Autodesk Inventor part; units mm, degrees
ref_plane "YZ Plane" through (0, 0, 0) normal (1, 0, 0) x (0, 1, 0)
ref_plane "XZ Plane" through (0, 0, 0) normal (0, 1, 0) x (-1, 0, 0)
ref_plane "XY Plane" through (0, 0, 0) normal (0, 0, 1) x (1, 0, 0)
sketch "Sketch1" plane through (0, 0, 0) normal (0, 0, 1) x (1, 0, 0)
  line L0 (0, 0) -> (34.66, 0)
  line L1 (34.66, 0) -> (34.66, -34.66)
  line L2 (34.66, -34.66) -> (0, -34.66)
  line L3 (0, -34.66) -> (0, 0)
  dimension "d0" = 34.66
  dimension "d1" = 34.66
extrude "Extrusion1" add sketch "Sketch1" along normal blind 21.5
sketch "Sketch2" plane through (0, 0, 21.5) normal (0, 0, 1) x (1, 0, 0)
  line L0 (0, 0) -> (0, -34.66)
  line L1 (3, -3) -> (31.66, -3)
  line L2 (31.66, -3) -> (31.66, -31.66)
  line L3 (31.66, -31.66) -> (3, -31.66)
  line L4 (3, -31.66) -> (3, -3)
  line L5 (34.66, 0) -> (0, 0)
  line L6 (0, -34.66) -> (34.66, -34.66)
  line L7 (34.66, 0) -> (34.66, -34.66)
  dimension "d8" = 3
  dimension "d9" = 3
  dimension "d10" = 3
  dimension "d11" = 3
extrude "Extrusion2" cut sketch "Sketch2" against normal blind 3.5 contours L1 L2 L3 L4
sketch "Sketch3" plane through (0, 0, 18) normal (0, 0, 1) x (1, 0, 0)
  line L0 (12.08, -3) -> (12.08, -6)
  line L1 (12.08, -6) -> (22.58, -6)
  line L2 (22.58, -6) -> (22.58, -3)
  line L3 (12.08, -3) -> (22.58, -3)
  line L4 (3, -3) -> (31.66, -3)
  line L5 (3, -31.66) -> (3, -3)
  line L6 (31.66, -3) -> (31.66, -31.66)
  line L7 (31.66, -31.66) -> (3, -31.66)
  point P0 (0, 0)
  dimension "d18" = 9.08
  dimension "d19" = 9.08
  dimension "d20" = 3
  dimension "d21" = 28.66
extrude "Extrusion3" cut sketch "Sketch3" against normal blind 19 contours L3 L2 L1 L0
properties part number "Pantalla"
Here's how the part is built. I have some questions about the finished solid (model axes, mm). A direction names the side the tool comes from. Round coordinates to 2 decimals unless told otherwise and drop trailing zeros. Order: outer loops, then holes, each group sorted by start corner. A loop starts at its lowest first (then second) coordinate and runs counter-clockwise, first axis right, second up. Notation, with made-up numbers: (-2.5, 50) -> (23.5, 50) arc R11 cw to (23.5, 66) -> close; hole circle Ø2 at (-1.5, -29.75). An arc over 180 degrees is marked (long way). Use a Markdown table: item, result. Add a question column.
(1) Suppose I cut it at B-B, the plane x = 13. Please give me the cut outline in (y, z).
(2) Suppose I cut it at D-D, the plane y = -26. Please give me the cut outline in (x, z).
(3) If we mould it in two halves opening along Y, with no side actions, what happens to faces 1 (the face through (22.58, -5, 9)), 2 (the face through (17, 0, 11)), 3 (the face through (34.66, -17, 11))? For each: released by +Y, released by -Y, zero draft, split by the parting line, or undercut.
(4) I need wall thicknesses on line 1 along X through (y, z) = (-5, 3); line 2 along Y through (x, z) = (20, 8.25); line 3 along Z through (x, y) = (11, -4). Which ranges of each line are inside material? Lowest first, please.
(5) For faces 4 (the face through (0, -18, 11)), 5 (the face through (17, -6, 9)), 6 (the face through (31.66, -17, 20)), which set-ups out of +Z, -Z, +X, -X, +Y, -Y let a thin tool reach every point of the face, with its end or its side?
(6) Suppose I cut it at C-C, the plane z = 9.75. Please give me the cut outline in (x, y).
(7) Suppose I cut it at A-A, the plane y = -5. Please give me the cut outline in (x, z).
(8) For pin 1 Ø1 at (x, y) = (12.5, -8.5) entering from +Z, with a flat end and sliding along its axis, tell me the tip position at first contact or that it passes through.
Verdict:
| question | item | result |
|---|---|---|
| 1 | outline | (-34.66, 0) -> (-6, 0) -> (-6, 18) -> (-31.66, 18) -> (-31.66, 21.5) -> (-34.66, 21.5) -> close; (-3, 0) -> (0, 0) -> (0, 21.5) -> (-3, 21.5) -> close |
| 2 | outline | (0, 0) -> (34.66, 0) -> (34.66, 21.5) -> (31.66, 21.5) -> (31.66, 18) -> (3, 18) -> (3, 21.5) -> (0, 21.5) -> close |
| 3 | face 1 | undercut |
| 3 | face 2 | released by +Y |
| 3 | face 3 | zero draft |
| 4 | line 1 | 0 to 12.08, 22.58 to 34.66 |
| 4 | line 2 | -34.66 to -6, -3 to 0 |
| 4 | line 3 | 0 to 18 |
| 5 | face 4 | +Z, -Z, -X, +Y, -Y |
| 5 | face 5 | +Z, -Z |
| 5 | face 6 | +Z |
| 6 | outline | (0, -34.66) -> (34.66, -34.66) -> (34.66, 0) -> (0, 0) -> close; hole (12.08, -6) -> (22.58, -6) -> (22.58, -3) -> (12.08, -3) -> close |
| 7 | outline | (0, 0) -> (12.08, 0) -> (12.08, 18) -> (3, 18) -> (3, 21.5) -> (0, 21.5) -> close; (22.58, 0) -> (34.66, 0) -> (34.66, 21.5) -> (31.66, 21.5) -> (31.66, 18) -> (22.58, 18) -> close |
| 8 | pin 1 | z = 18 |
